Input: dimensioned drawing with shaded views. Units: mm. Origin: part minimum x, y, z. A direction names the side the tool comes from. Round coordinates to 2 decimals unless told otherwise and drop trailing zeros. Order: outer loops, then holes, each group sorted by start corner. A loop starts at its lowest first (then second) coordinate and runs counter-clockwise, first axis right, second up. Notation, with made-up numbers: M -28.5,-11.5 L -0.5,-11.5 A21 cw -0.5,-7.5 Z; hole C 64,70.5 d10. An arc over 180 degrees is marked long. Use one line per item in the form item = value. Start each with the question number.
Q1. Section B-B (x = 112.5). Return the cut outline in (y, z).
Q2. Reachability of the marked faces 1 and 2 from +Z, -Z, +X, -X, +Y, -Y: full face, straight path, thin tool, end or side. Return the list, or none.
Q3. Section C-C (y = 5). Give the number of separate pieces and of enclosed holes in the cut face, plus the area to 3 significant figures.
Q4. Contact query for flat-ended pins moving along their axis: pin 1 (5 mm diameter, centred on x = 96.5, y = 10.5, fed in from -Z); pin 2 (17 mm diameter, centred on x = 23.54, z = 61.36, fed in from +Y); pin 3 (8 mm diameter, centred on y = 7.5, z = 146, fed in from -X). Output: stop coordinate, or through.
Q5. Section A-A (z = 10). Return the cut outline in (x, y).
Q6. Material intervals for probe 1 along Z at (x, y) = (113, 11); probe 2 along Z at (x, y) = (202.5, 1.5) (1 decimal); probe 3 along X at (y, z) = (5, 164.5) (1 decimal), sorted ascending.
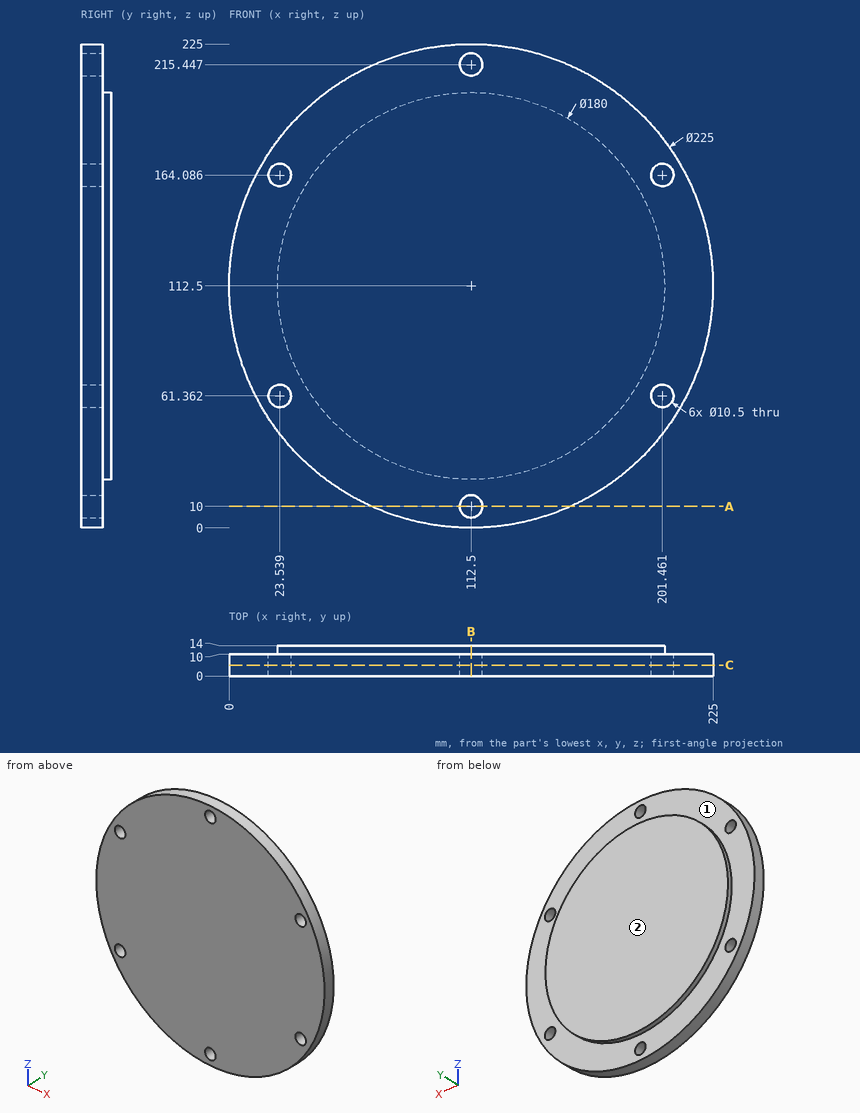
Results list:
q1.outline = M 0,0 L 10,0 L 10,4.75 L 0,4.75 Z; M 0,15.25 L 10,15.25 L 10,22.5 L 14,22.5 L 14,202.5 L 10,202.5 L 10,210.2 L 0,210.2 Z; M 0,220.7 L 10,220.7 L 10,225 L 0,225 Z
q2.face_1 = +Y
q2.face_2 = +Z, -Z, +X, -X, +Y
q3.separate_pieces = 1
q3.enclosed_holes = 6
q3.area = 39,200 mm2
q4.pin_1 = 0.82
q4.pin_2 = 10
q4.pin_3 = 3.94
q5.outline = M 66.13,0 L 107.25,0 L 107.25,10 L 66.13,10 Z; M 117.75,0 L 158.87,0 L 158.87,10 L 117.75,10 Z
q6.probe_1 = 22.5 to 202.5
q6.probe_2 = 45 to 56.2, 66.5 to 158.9, 169.2 to 180
q6.probe_3 = 12.7 to 18.3, 28.8 to 196.2, 206.7 to 212.3
